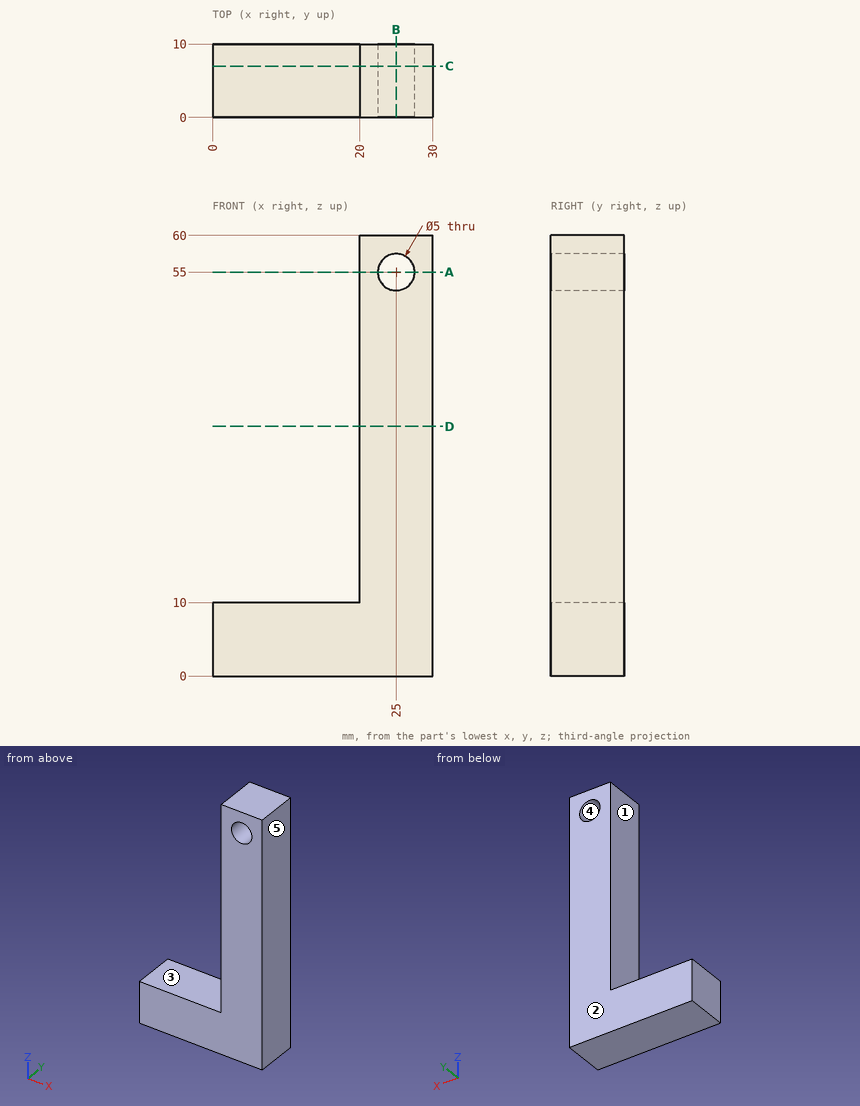
Verification items for this drawing (mm, ordinates from the low corner). A direction names the side the tool comes from. Give positions to 0.01 mm unless a question says otherwise; leave off trailing zeros. Write each loop counter-clockwise with the first axis right and the second up, starting at its lowest first coordinate (ties: lowest second). Pieces come first, ordered by that corner, then holes.
1) Cross-section at B-B (x = 25). Record the boundary of the cut face in (y, z), plus the area to 3 significant figures.
Values follow:
outline: (0, 0) - (10, 0) - (10, 52.5) - (0, 52.5) - close; (0, 57.5) - (10, 57.5) - (10, 60) - (0, 60) - close
area: 550 mm2
2) Go/stop test with a flat-tipped pin: pin 1 Ø2 at (y, z) = (6, 36.5) entering from -X. Record where the tip stops, or that it passes through.
Values follow:
pin 1: stops at x = 20
3) Cross-section at A-A (z = 55). Record the boundary of the cut face in (x, y).
Values follow:
outline: (20, 0) - (22.5, 0) - (22.5, 10) - (20, 10) - close; (27.5, 0) - (30, 0) - (30, 10) - (27.5, 10) - close
4) Thickness scan on line 1 (Z direction, x = 25, y = 3); line 2 (Z direction, x = 6, y = 9.5); line 3 (X direction, y = 1.5, z = 28). Record the ranges inside material, lowest first.
Values follow:
line 1: z = 0 to 52.5, 57.5 to 60
line 2: z = 0 to 10
line 3: x = 20 to 30
5) Release check for a two-part mould opening along Z. For the marked faces 3, 4 and 5 record: released by +Z, released by -Z, zero draft, split by the parting line, or undercut.
Values follow:
face 3: released by +Z
face 4: undercut
face 5: zero draft
6) Set-up check for the marked faces 1 and 2: record each of +Z, -Z, +X, -X, +Y, -Y from which the full face is reachable in a straight line by a thin tool's end or side.
Values follow:
face 1: +Z, -X, +Y, -Y
face 2: +Z, -Z, +X, -X, +Y
7) Cross-section at D-D (z = 34). Record the boundary of the cut face in (x, y), plus the area to 3 significant figures.
Values follow:
outline: (20, 0) - (30, 0) - (30, 10) - (20, 10) - close
area: 100 mm2
8) Cross-section at C-C (y = 7). Record the boundary of the cut face in (x, z), plus the area to 3 significant figures.
Values follow:
outline: (0, 0) - (30, 0) - (30, 60) - (20, 60) - (20, 10) - (0, 10) - close; hole circle Ø5 at (25, 55)
area: 780 mm2
